Read the model definition and answer for the solid it produces. Units are mm, in the model's axes. Face numbers are marked on the shaded views. A direction names the side the tool comes from. Coordinates: 2 decimals unless noted, no trailing zeros. Write each loop counter-clockwise with the first axis right and the second up, starting at its lowest first coordinate (ties: lowest second). Pieces come first, ordered by that corner, then holes.
(1) Section B-B on x = 0 is taken. Write down the section's boundary in (y, z) (3 decimals), then the cut area to 3 significant figures.
(2) The mould has two halves that part along Z. Classify the marked faces 1, 2 and 3: +Z half, -Z half, draft (parallel to the pull), parting line (faces both ways), or undercut.
(3) Section A-A on z = 0 is taken. Write down the section's boundary in (x, y) (3 decimals), then the cut area to 3 significant figures.
(4) Which of the six approach directions +Z, -Z, +X, -X, +Y, -Y give full straight-line access (tool end or side, diameter ignored) to the marked faces 4, 5, 6 and 7?
(5) Find the intervals of material crossed by probe 1 along Y at (x, z) = (-16, -78); probe 2 along X at (y, z) = (-15, -77); probe 3 along X at (y, z) = (-15, -55), in increasing order.
(6) Section D-D on x = -16 is taken. State how many separate pieces and enclosed holes the cut face has, then the cut area to 3 significant figures.
(7) Given pin 1 (1.2 mm diameter, centred on y = 28.5, z = -70, fed in from -X); pin 2 (0.5 mm diameter, centred on y = -29, z = -71.5, fed in from +X); pin 3 (12 mm diameter, centred on x = -48, y = 6, fed in from +Z), each flat-ended and moving along its own axis, determine where each tip first touches the part or whether it passes through.
(8) Section C-C on y = -6 is taken. Write down the section's boundary in (x, z) (3 decimals), then the cut area to 3 significant figures.
from build123d import *

# Parameters (mm, degrees)
SKETCH1_W                                       = 12
SKETCH1_H                                       = 18
BOSS_EXTRUDE1_DEPTH                             = 29.25
SKETCH4_W                                       = 45
SKETCH4_H                                       = 10
BOSS_EXTRUDE2_DEPTH                             = 4.5
CSK_FOR_M5_FLAT_HEAD_MACHINE_SCREW1_AT_2_COUNT  = 2
CSK_FOR_M5_FLAT_HEAD_MACHINE_SCREW1_AT_2_PITCH  = 32
CSK_FOR_M5_FLAT_HEAD_MACHINE_SCREW1_AT_3_COUNT  = 2
CSK_FOR_M5_FLAT_HEAD_MACHINE_SCREW1_AT_3_PITCH  = 43.863424399
CSK_FOR_M5_FLAT_HEAD_MACHINE_SCREW1_AT_4_COUNT  = 2
CSK_FOR_M5_FLAT_HEAD_MACHINE_SCREW1_AT_4_PITCH  = 30
CUT_EXTRUDE1_REACH                              = 137.259
CUT_EXTRUDE1_END_RADIUS                         = 57.15
SKETCH13_R                                      = 5.2
CHAMFER1_SIZE                                   = 3.556619638
CHAMFER1_SIZE_2                                 = 3.175
CHAMFER2_SIZE                                   = 1
CSK_FOR_M3_FLAT_HEAD_MACHINE_SCREW1_D           = 3.4
CSK_FOR_M3_FLAT_HEAD_MACHINE_SCREW1_DEPTH       = 15
CSK_FOR_M3_FLAT_HEAD_MACHINE_SCREW1_CSINK_D     = 6.3
CSK_FOR_M3_FLAT_HEAD_MACHINE_SCREW1_CSINK_ANGLE = 90
CSK_FOR_M3_FLAT_HEAD_MACHINE_SCREW1_TIP         = 1.021463052
SKETCH17_R                                      = 4
CUT_EXTRUDE2_DEPTH                              = 17.5
CUT_EXTRUDE3_START                              = -4
CUT_EXTRUDE3_DEPTH                              = 10


with BuildPart() as part:
    # Sketch1 → Boss-Extrude1 (new, symmetric)
    with BuildSketch(Plane(origin=(0, 0, 0), x_dir=(1, 0, 0), z_dir=(0, 1, 0))):
        with BuildLine():
            Line((-27.5, 53.692230583), (-27.5, 93.692230583))
            Line((-27.5, 93.692230583), (-22.5, 93.692230583))
            Line((-22.5, 93.692230583), (-22.5, 83.692230583))
            Line((-22.5, 83.692230583), (22.5, 83.692230583))
            Line((22.5, 83.692230583), (22.5, 93.692230583))
            Line((22.5, 93.692230583), (32.5, 93.692230583))
            Line((32.5, 93.692230583), (32.5, 68.433749194))
            Line((32.5, 68.433749194), (37.690810999, 64.078141599))
            Line((37.690810999, 64.078141599), (29.139173324, 53.886696677))
            Line((29.139173324, 53.886696677), (32.96939554, 50.672758629))
            Line((32.96939554, 50.672758629), (41.521033215, 60.864203551))
            Line((41.521033215, 60.864203551), (45.351255431, 57.650265502))
            Line((45.351255431, 57.650265502), (36.799617755, 47.45882058))
            Line((36.799617755, 47.45882058), (38.801277269, 41.959306266))
            ThreePointArc((38.801277269, 41.959306266), (-40.514490328, -40.307549832), (42.157451983, 38.585900823))
            Line((42.157451983, 38.585900823), (39.655856522, 45.458977865))
            Line((39.655856522, 45.458977865), (48.012095448, 55.417555625))
            Line((48.012095448, 55.417555625), (51.842317663, 52.203617577))
            Line((51.842317663, 52.203617577), (43.290679988, 42.012172655))
            ThreePointArc((43.290679988, 42.012172655), (-9.820505686, -59.520276319), (-27.5, 53.692230583))
        make_face()
        with Locations((0, 70.421115292)):
            Rectangle(SKETCH1_W, SKETCH1_H, mode=Mode.SUBTRACT)
    extrude(amount=BOSS_EXTRUDE1_DEPTH, both=True)

    # Sketch4 → Boss-Extrude2 (add)
    with BuildSketch(Plane.XZ.offset(29.25)):
        with Locations((0, -88.692230583)):
            Rectangle(SKETCH4_W, SKETCH4_H)
    extrude(amount=-BOSS_EXTRUDE2_DEPTH)

    # Sketch12 → CSK for M5 Flat Head Machine Screw1 (revolve, cut)
    with BuildSketch(Plane(origin=(-16, 15, -57.15), x_dir=(0, -1, 0), z_dir=(1, 0, 0))):
        Polygon((0, 0), (0, 36.542230583), (2.75, 36.542230583), (2.75, 2.45), (5.2, 0), align=None)
    csk_for_m5_flat_head_machine_screw1 = revolve(axis=Axis((-16, 15, -50.8), (0, 0, -1)), mode=Mode.SUBTRACT)

    # CSK for M5 Flat Head Machine Screw1 at 2: CSK for M5 Flat Head Machine Screw1 ×2
    with Locations(*[(i * CSK_FOR_M5_FLAT_HEAD_MACHINE_SCREW1_AT_2_PITCH, 0, 0) for i in range(1, CSK_FOR_M5_FLAT_HEAD_MACHINE_SCREW1_AT_2_COUNT)]):
        add(csk_for_m5_flat_head_machine_screw1, mode=Mode.SUBTRACT)

    # CSK for M5 Flat Head Machine Screw1 at 3: CSK for M5 Flat Head Machine Screw1 ×2
    with Locations(*[Vector(0.7295372041400852, -0.6839411288813297, 0) * (i * CSK_FOR_M5_FLAT_HEAD_MACHINE_SCREW1_AT_3_PITCH) for i in range(1, CSK_FOR_M5_FLAT_HEAD_MACHINE_SCREW1_AT_3_COUNT)]):
        add(csk_for_m5_flat_head_machine_screw1, mode=Mode.SUBTRACT)

    # CSK for M5 Flat Head Machine Screw1 at 4: CSK for M5 Flat Head Machine Screw1 ×2
    with Locations(*[(0, -i * CSK_FOR_M5_FLAT_HEAD_MACHINE_SCREW1_AT_4_PITCH, 0) for i in range(1, CSK_FOR_M5_FLAT_HEAD_MACHINE_SCREW1_AT_4_COUNT)]):
        add(csk_for_m5_flat_head_machine_screw1, mode=Mode.SUBTRACT)

    # Cut-Extrude1: up to this cylinder (the profile starts outside it)
    cut_extrude1_end = Plane(origin=(0, 0, 0), z_dir=(0, -1, 0)) * Cylinder(CUT_EXTRUDE1_END_RADIUS, 419.818, mode=Mode.PRIVATE)
    # Sketch13 → Cut-Extrude1 (cut, up to the surface)
    with BuildSketch(Plane.XY.offset(-57.15), mode=Mode.PRIVATE) as cut_extrude1_sk1:
        with Locations(Location((-16, -15, 0), (0, 0, 180))):
            Circle(SKETCH13_R)
    cut_extrude1_tool1 = extrude(cut_extrude1_sk1.sketch, amount=CUT_EXTRUDE1_REACH, mode=Mode.PRIVATE) - cut_extrude1_end
    add(cut_extrude1_tool1.solids().sort_by_distance((-16, -15, -57.15))[0], mode=Mode.SUBTRACT)
    # Sketch13 → Cut-Extrude1 (cut, up to the surface)
    with BuildSketch(Plane.XY.offset(-57.15), mode=Mode.PRIVATE) as cut_extrude1_sk2:
        with Locations(Location((16, -15, 0), (0, 0, 180))):
            Circle(SKETCH13_R)
    cut_extrude1_tool2 = extrude(cut_extrude1_sk2.sketch, amount=CUT_EXTRUDE1_REACH, mode=Mode.PRIVATE) - cut_extrude1_end
    add(cut_extrude1_tool2.solids().sort_by_distance((16, -15, -57.15))[0], mode=Mode.SUBTRACT)
    # Sketch13 → Cut-Extrude1 (cut, up to the surface)
    with BuildSketch(Plane.XY.offset(-57.15), mode=Mode.PRIVATE) as cut_extrude1_sk3:
        with Locations(Location((16, 15, 0), (0, 0, 180))):
            Circle(SKETCH13_R)
    cut_extrude1_tool3 = extrude(cut_extrude1_sk3.sketch, amount=CUT_EXTRUDE1_REACH, mode=Mode.PRIVATE) - cut_extrude1_end
    add(cut_extrude1_tool3.solids().sort_by_distance((16, 15, -57.15))[0], mode=Mode.SUBTRACT)
    # Sketch13 → Cut-Extrude1 (cut, up to the surface)
    with BuildSketch(Plane.XY.offset(-57.15), mode=Mode.PRIVATE) as cut_extrude1_sk4:
        with Locations(Location((-16, 15, 0), (0, 0, 180))):
            Circle(SKETCH13_R)
    cut_extrude1_tool4 = extrude(cut_extrude1_sk4.sketch, amount=CUT_EXTRUDE1_REACH, mode=Mode.PRIVATE) - cut_extrude1_end
    add(cut_extrude1_tool4.solids().sort_by_distance((-16, 15, -57.15))[0], mode=Mode.SUBTRACT)

    # Chamfer1
    # the kernel refuses this chamfer: 7.31254539, 3.556619638, 3.175 mm, written as the material it adds along each edge
    with BuildSketch(Plane(origin=(43.290679988, -29.25, -42.012172655), x_dir=(0.6767582135890655, 0, 0.736205352017857), z_dir=(0, 1, 0))) as chamfer1_piece_1:
        with BuildLine():
            Line((3.264526209, 0), (-CHAMFER1_SIZE * 0.128954224472, CHAMFER1_SIZE * 0.99165054742))
            Line((-CHAMFER1_SIZE * 0.128954224472, CHAMFER1_SIZE * 0.99165054742), (0, 0))
            ThreePointArc((0, 0), (1.683964682, 0.02206463), (3.264526209, 0))
        make_face()
    extrude(amount=58.5)
    with BuildSketch(Plane(origin=(-27.5, -29.25, -53.692230583), x_dir=(0, 0, -1), z_dir=(0, 1, 0))) as chamfer1_piece_2:
        with BuildLine():
            Line((CHAMFER1_SIZE_2, 0), (-5.17652137, 8.35152137))
            ThreePointArc((-5.17652137, 8.35152137), (-2.493388985, 4.40273098), (0, 0))
            Line((0, 0), (CHAMFER1_SIZE_2, 0))
        make_face()
    extrude(amount=58.5)

    # Chamfer2
    chamfer2_edges = [part.edges().sort_by_distance(p)[0] for p in [
        (29.139173324, 0, -53.886696677),
        (32.96939554, 0, -50.672758629),
    ]]
    chamfer(chamfer2_edges, length=CHAMFER2_SIZE)

    # CSK for M3 Flat Head Machine Screw1
    with Locations(Plane(origin=(4.717057163, 0, 3.958080926), x_dir=(0.6427876096865344, 0, -0.7660444431189822), z_dir=(0.7660444431189822, 0, 0.6427876096865344))):
        with Locations((68.440207181, 20), (68.440207181, 0), (68.440207181, -20)):
            CounterSinkHole(CSK_FOR_M3_FLAT_HEAD_MACHINE_SCREW1_D / 2, CSK_FOR_M3_FLAT_HEAD_MACHINE_SCREW1_CSINK_D / 2, depth=CSK_FOR_M3_FLAT_HEAD_MACHINE_SCREW1_DEPTH, counter_sink_angle=CSK_FOR_M3_FLAT_HEAD_MACHINE_SCREW1_CSINK_ANGLE)
            with Locations((0, 0, -(CSK_FOR_M3_FLAT_HEAD_MACHINE_SCREW1_DEPTH + CSK_FOR_M3_FLAT_HEAD_MACHINE_SCREW1_TIP / 2))):  # 118° drill point
                Cone(0, CSK_FOR_M3_FLAT_HEAD_MACHINE_SCREW1_D / 2, CSK_FOR_M3_FLAT_HEAD_MACHINE_SCREW1_TIP, mode=Mode.SUBTRACT)

    # Sketch17 → Cut-Extrude2 (cut)
    with BuildSketch(Plane.ZY.offset(27.5)):
        with Locations((-70.421115292, 31.25)):
            Circle(SKETCH17_R)
    cut_extrude2 = extrude(amount=-CUT_EXTRUDE2_DEPTH, mode=Mode.SUBTRACT)

    # Sketch19 → Cut-Extrude3 (cut)
    with BuildSketch(Plane.ZY.offset(-6).offset(CUT_EXTRUDE3_START)):
        Polygon((-68.400389349, 34.75), (-72.441841234, 34.75), (-74.462567176, 31.25), (-72.441841234, 27.75), (-68.400389349, 27.75), (-66.379663407, 31.25), align=None)
    cut_extrude3 = extrude(amount=-CUT_EXTRUDE3_DEPTH, mode=Mode.SUBTRACT)

    # Mirror1: Cut-Extrude2, Cut-Extrude3 across plane
    add(cut_extrude2.mirror(Plane.ZX), mode=Mode.SUBTRACT)
    add(cut_extrude3.mirror(Plane.ZX), mode=Mode.SUBTRACT)


solid = part.part
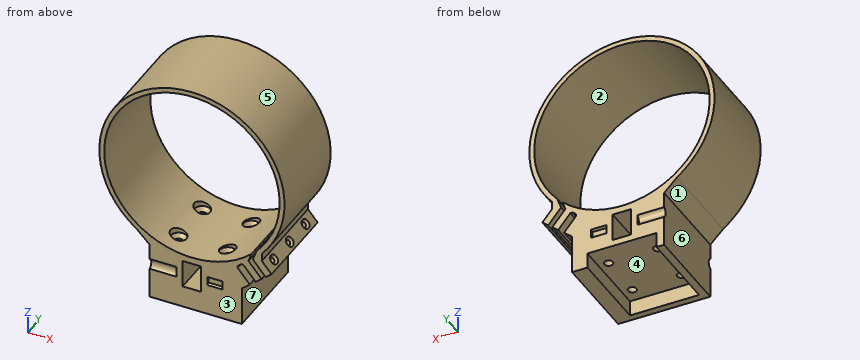
Response:
1. outline: (-29.25, -93.692) - (-24.75, -93.692) - (-24.75, -83.692) - (29.25, -83.692) - (29.25, -79.421) - (-29.25, -79.421) - close; (-29.25, -61.421) - (29.25, -61.421) - (29.25, -57.15) - (-29.25, -57.15) - close; (-29.25, 57.15) - (29.25, 57.15) - (29.25, 60.325) - (-29.25, 60.325) - close
1. area: 730 mm2
2. face 1: -Z half
2. face 2: undercut
2. face 3: draft
3. outline: (-60.325, -29.25) - (-57.15, -29.25) - (-57.15, 29.25) - (-60.325, 29.25) - close; (57.15, -29.25) - (60.325, -29.25) - (60.325, 29.25) - (57.15, 29.25) - close
3. area: 371 mm2
4. face 4: -Z, +Y
4. face 5: +Y, -Y
4. face 6: -Z, -X, +Y, -Y
4. face 7: -Z, +X, +Y, -Y
5. probe 1: y = -29.25 to -17.75, -12.25 to 12.25, 17.75 to 29.25
5. probe 2: x = -27.5 to -18.75, -13.25 to -6, 6 to 13.25, 18.75 to 32.5
5. probe 3: x = -29.37 to -21.2, 21.2 to 30.07, 36.6 to 43.13, 47.66 to 48.51
6. separate pieces: 4
6. enclosed holes: 0
6. area: 1,550 mm2
7. pin 1: stops at x = -10
7. pin 2: stops at x = 32.5
7. pin 3: stops at z = 43.3
8. outline: (-35.852, -48.516) - (-27.5, -56.867) - (-27.5, -93.692) - (-22.5, -93.692) - (-22.5, -83.692) - (22.5, -83.692) - (22.5, -93.692) - (32.5, -93.692) - (32.5, -68.434) - (37.691, -64.078) - (29.782, -54.653) - (29.905, -53.244) - (32.203, -51.316) - (33.612, -51.439) - (41.521, -60.864) - (45.351, -57.65) - (36.8, -47.459) - (38.801, -41.959) arc R57.15 cw (long way) to (42.157, -38.586) - (39.656, -45.459) - (48.012, -55.418) - (51.842, -52.204) - (45.577, -44.737) - (45.5, -39.609) arc R60.325 ccw (long way) to start; hole (-6, -79.421) - (6, -79.421) - (6, -61.421) - (-6, -61.421) - close
8. area: 2,820 mm2
